from build123d import *

# Parameters (mm, degrees)
SKETCH5_W          = 40
SKETCH5_H          = 10
CUT_EXTRUDE3_DEPTH = 45
SKETCH6_R          = 2.75
CUT_EXTRUDE4_DEPTH = 45


with BuildPart() as part:
    # Sketch4 → Revolve2 (revolve)
    with BuildSketch(Plane(origin=(0, 0, 0), x_dir=(0, 0, -1), z_dir=(1, 0, 0))):
        Polygon((22, 11), (12, 11), (12, 8), (-12, 8), (-12, 11), (-22, 11), (-22, 24), (-12, 24), (-12, 14), (22, 14), align=None)
    revolve(axis=Axis((0, 0, 17.928277082), (0, 0, -1)))

    # Sketch5 → Cut-Extrude3 (cut, through all)
    with BuildSketch(Plane.XY.offset(22)):
        with Locations((0, 25)):
            Rectangle(SKETCH5_W, SKETCH5_H)
        with Locations((0, -25)):
            Rectangle(SKETCH5_W, SKETCH5_H)
    extrude(amount=-CUT_EXTRUDE3_DEPTH, mode=Mode.SUBTRACT)

    # Sketch6 → Cut-Extrude4 (cut, through all)
    with BuildSketch(Plane.XY.offset(22)):
        with Locations((-19, 0)):
            Circle(SKETCH6_R)
        with Locations((-13.435028843, 13.435028843)):
            Circle(SKETCH6_R)
        with Locations((13.435028843, 13.435028843)):
            Circle(SKETCH6_R)
        with Locations((19, 0)):
            Circle(SKETCH6_R)
        with Locations((13.435028843, -13.435028843)):
            Circle(SKETCH6_R)
        with Locations((-13.435028843, -13.435028843)):
            Circle(SKETCH6_R)
    extrude(amount=-CUT_EXTRUDE4_DEPTH, mode=Mode.SUBTRACT)


solid = part.part
For this review, take the finished solid that the model builds, in its own axes (mm). A direction names the side the tool comes from. Give positions to 0.01 mm unless a question says otherwise; leave off trailing zeros. Loops run counter-clockwise (first coordinate to the right, second up) from the corner with the lowest first, then second, coordinate; pieces in that order, holes last. Notation, with made-up numbers: M -36,0 L -15,0 A11 cw -15,17 Z; hole C 83,48.25 d4. An arc over 180 degrees is marked long. Put each result on its own line as item: value. Start each with the question number.
(1) Add section B-B, the plane y = 0. Write out the cut boundary in (x, z).
(2) Add section A-A, the plane x = 0. Write out the cut boundary in (y, z).
(3) Add section C-C, the plane y = 5. Write out the cut boundary in (x, z) (3 decimals), then the cut area to 3 significant figures.
(4) For pin 1 (2 mm diameter, centred on x = 8.5, z = 10, fed in from -Y); pin 2 (12 mm diameter, centred on y = 8, z = 14.5, fed in from -X); pin 3 (1.5 mm diameter, centred on y = -2, z = 5, fed in from +X), all flat-tipped, find the tip position at first contact; note any pin that passes through.
(5) Machinability: for faces 1 (the cylindrical face through (-24, 0, 17)), 2 (the flat face through (-8, -2, -12)), 3 (the flat face through (-8, 2, 12)), which of the approach directions +Z, -Z, +X, -X, +Y, -Y give a long, thin tool a straight path to every point of the face, cutting with its end or side? Answer none if there is none.
(6) The part is to be moulded in two halves that separate along Y. For faces 4 (the cylindrical face through (16.253, 0.121, 17.07)), 5 (the flat face through (-9.3, 6.2, -22)), 6 (the flat face through (0, -20, 17)), say which applies: +Y half, -Y half, draft (parallel to the pull), parting line (faces both ways), or undercut.
(7) Add section D-D, the plane z = -1.5. Write out the cut boundary in (x, y).
(8) Wall thickness on L1, parallel to X at y = 0, z = 6.75; L2, parallel to Y at x = 0.5, z = -4; L3, parallel to Z at x = 10.5, y = 0.5: over which ranges is each line inside the solid? List them lowest first.
Result:
1. outline: M -24,12 L -21.75,12 L -21.75,22 L -24,22 Z; M -16.25,12 L -14,12 L -14,-22 L -11,-22 L -11,-12 L -8,-12 L -8,12 L -11,12 L -11,22 L -16.25,22 Z; M 8,-12 L 11,-12 L 11,-22 L 14,-22 L 14,12 L 16.25,12 L 16.25,22 L 11,22 L 11,12 L 8,12 Z; M 21.75,12 L 24,12 L 24,22 L 21.75,22 Z
2. outline: M -20,12 L -14,12 L -14,-22 L -11,-22 L -11,-12 L -8,-12 L -8,12 L -11,12 L -11,22 L -20,22 Z; M 8,-12 L 11,-12 L 11,-22 L 14,-22 L 14,12 L 20,12 L 20,22 L 11,22 L 11,12 L 8,12 Z
3. outline: M -23.473,12 L -13.077,12 L -13.077,-22 L -9.798,-22 L -9.798,-12 L -6.245,-12 L -6.245,12 L -9.798,12 L -9.798,22 L -23.473,22 Z; M 6.245,-12 L 9.798,-12 L 9.798,-22 L 13.077,-22 L 13.077,12 L 23.473,12 L 23.473,22 L 9.798,22 L 9.798,12 L 6.245,12 Z
3. area: 667 mm^2
4. pin 1: stops at y = -11.82
4. pin 2: stops at x = -23.92
4. pin 3: stops at x = 13.94
5. face 1: +Z, -Z, -X
5. face 2: -Z
5. face 3: +Z
6. face 4: undercut
6. face 5: draft
6. face 6: -Y half
7. outline: C 0,0 d28; hole C 0,0 d16
8. L1: x = -14 to -8, 8 to 14
8. L2: y = -13.99 to -7.98, 7.98 to 13.99
8. L3: z = -12 to 12
